Drawing for the job (mm, zero at the part's lowest x, y, z). A direction names the side the tool comes from. Round coordinates to 2 decimals unless told otherwise and drop trailing zeros. Use a Markdown table: item, result.
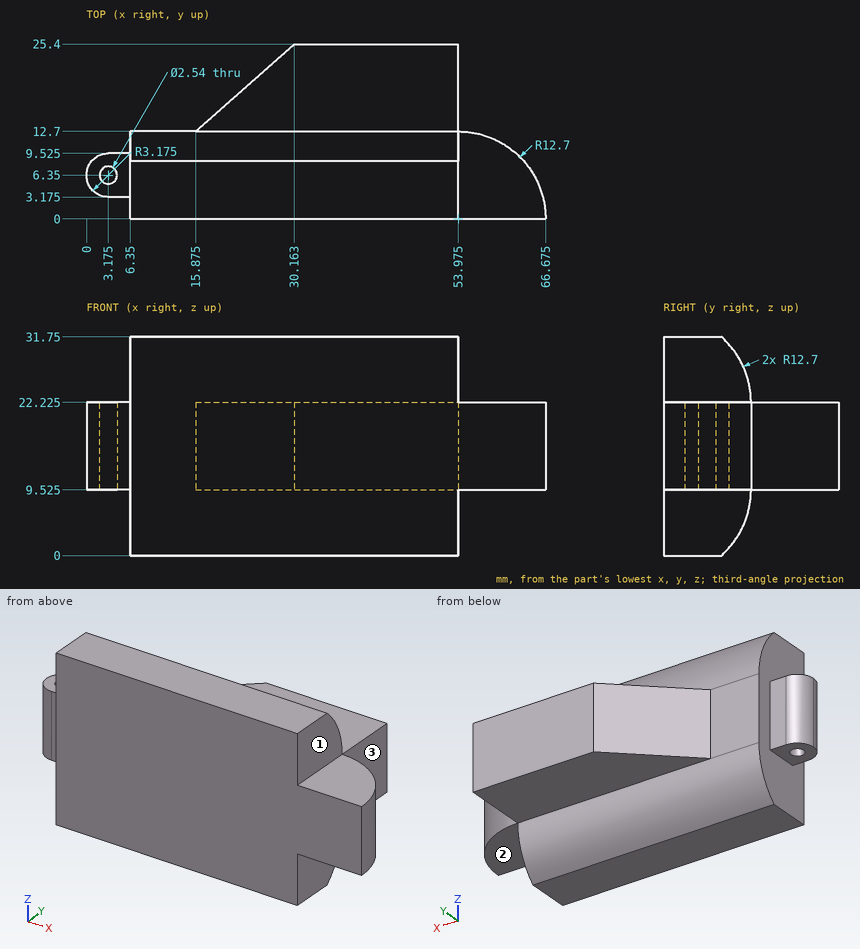
Q1. Drop flat-ended pins along their axis: P1, Ø1, axis at x = 5, z = 16, coming from the +Y side (1 decimal); P2, Ø1, axis at x = 50, z = 25, coming from the +Y side (1 decimal); P3, Ø10, axis at y = 19.5, z = 16, coming from the +X side (1 decimal). Give the stop position or say it passes through.
Response values:
| item | result |
|---|---|
| P1 | stops at y = 9.5 |
| P2 | stops at y = 12.5 |
| P3 | stops at x = 54 |
Q2. Drill centre lines: L1, parallel to Y at x = 45, z = 9; L2, parallel to Y at x = 63.5, z = 10.5; L3, parallel to Z at x = 45, y = 23.25 (1 decimal). Where is each one in solid material? Low to high.
Response values:
| item | result |
|---|---|
| L1 | y = 0 to 12.69 |
| L2 | y = 0 to 8.4 |
| L3 | z = 9.5 to 22.2 |
Q3. Which spindle directions (+Z, -Z, +X, -X, +Y, -Y) get a long thin tool onto all of the face, cutting with end or side? Do the marked faces 1, 2 and 3. Say none if no direction does.
Response values:
| item | result |
|---|---|
| face 1 | +Z, +X, +Y, -Y |
| face 2 | -Z, +X, +Y, -Y |
| face 3 | +Z, -Z, +X, +Y |
